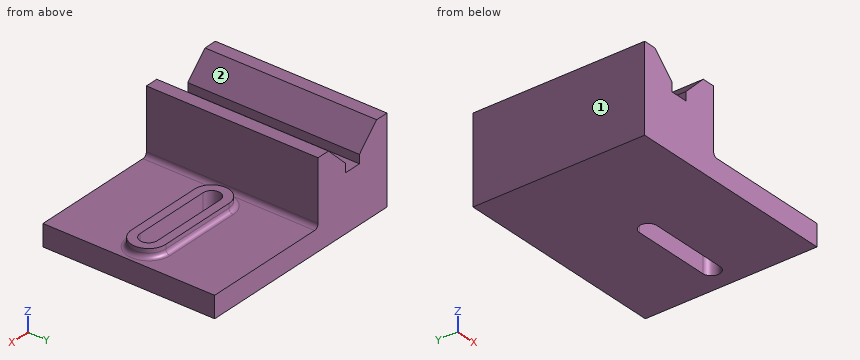
```python
from build123d import *

# Parameters (mm, degrees)
F1_DEPTH    = 200
F3_DEPTH    = 10
F4_DEPTH    = 25
F5_T1_DEPTH = 200
F5_T3_DEPTH = 91.5131680667
F5_T6_ANGLE = 180
F5_T8_ANGLE = 180


# Not quite as in the source:
# - a fillet or chamfer that OpenCascade refuses, or shapes differently, is made with other operations: its cross-section is extruded or revolved along the edge and cut away or added


with BuildPart() as f1:
    # F0 (on Front) → F1 (new body)
    with BuildSketch(Plane.XZ):
        Polygon((-250, 0), (0, 0), (0, 25), (-150, 25), (-150, 100), (-165, 100), (-190, 75), (-190, 65), (-210, 65), (-210, 75), (-235, 100), (-250, 100), align=None)
    extrude(amount=F1_DEPTH)

    # F2 (on face) → F3 (join)
    with BuildSketch(Plane.XY.offset(25)):
        with BuildLine():
            Line((-120.2453300357, -120), (-28.7321619689, -120))
            ThreePointArc((-28.7321619689, -120), (-8.7321619689, -100), (-28.7321619689, -80))
            Line((-28.7321619689, -80), (-120.2453300357, -80))
            ThreePointArc((-120.2453300357, -80), (-140.2453300357, -100), (-120.2453300357, -120))
        make_face()
        with BuildLine():
            ThreePointArc((-28.7321619689, -90), (-18.7321619689, -100), (-28.7321619689, -110))
            Line((-28.7321619689, -110), (-120.2453300357, -110))
            ThreePointArc((-120.2453300357, -110), (-130.2453300357, -100), (-120.2453300357, -90))
            Line((-120.2453300357, -90), (-28.7321619689, -90))
        make_face(mode=Mode.SUBTRACT)
    extrude(amount=F3_DEPTH)

    # F4 (cut): a face of the model
    f4_faces = [f1.faces().sort_by_distance(p)[0] for p in [
        (-74.4887460023, -100, 25),
    ]]
    extrude(f4_faces, amount=-F4_DEPTH, mode=Mode.SUBTRACT)

    # F5: fillet of radius 5 on 3 edges, made by hand

    # F5_s2 → F5_t1 (join)
    with BuildSketch(Plane.XZ):
        with BuildLine():
            ThreePointArc((-145, 25), (-148.5355339059, 26.4644660941), (-150, 30))
            Line((-150, 30), (-150, 25))
            Line((-150, 25), (-145, 25))
        make_face()
    extrude(amount=F5_T1_DEPTH)

    # F5_s4 → F5_t3 (join)
    with BuildSketch(Plane.YZ.offset(-120.2453300357)):
        with BuildLine():
            ThreePointArc((-125, 25), (-121.4644660941, 26.4644660941), (-120, 30))
            Line((-120, 30), (-120, 25))
            Line((-120, 25), (-125, 25))
        make_face()
        with BuildLine():
            ThreePointArc((-75, 25), (-78.5355339059, 26.4644660941), (-80, 30))
            Line((-80, 30), (-80, 25))
            Line((-80, 25), (-75, 25))
        make_face()
    extrude(amount=F5_T3_DEPTH)

    # F5_s5 → F5_t6 (revolve)
    with BuildSketch(Plane.YZ.offset(-28.7321619689)):
        with BuildLine():
            ThreePointArc((-120, 30), (-121.4644660941, 26.4644660941), (-125, 25))
            Line((-125, 25), (-120, 25))
            Line((-120, 25), (-120, 30))
        make_face()
    revolve(axis=Axis((-28.7321619689, -100, 25), (0, 0, 1)), revolution_arc=F5_T6_ANGLE)

    # F5_s7 → F5_t8 (revolve)
    with BuildSketch(Plane.YZ.offset(-120.2453300357)):
        with BuildLine():
            ThreePointArc((-75, 25), (-78.5355339059, 26.4644660941), (-80, 30))
            Line((-80, 30), (-80, 25))
            Line((-80, 25), (-75, 25))
        make_face()
    revolve(axis=Axis((-120.2453300357, -100, 25), (0, 0, 1)), revolution_arc=F5_T8_ANGLE)


solid = f1.part
```
Can you work these out from the model? Positions are in its coordinate system, mm. Face numbers are marked on the shaded views. A direction names the side the tool comes from. Give positions to 0.01 mm unless a question says otherwise; leave off trailing zeros. Loops run counter-clockwise (first coordinate to the right, second up) from the corner with the lowest first, then second, coordinate; pieces in that order, holes last. Notation, with made-up numbers: M 58,-31 L 85,-31 A18 cw 85,-20 Z; hole C 25,20 d11. An arc over 180 degrees is marked long. Use CSV: the item, a comma, the result in double quotes. Start each with the question number.
1. If I drill on L1, parallel to X at y = -85.5, z = 70; L2, parallel to X at y = -101, z = 32.5; L3, parallel to Z at x = -24.5, y = -63.5, over which ranges is the centre line in solid material (lowest first)?
2. On a 3-axis mill with a long thin cutter (end or side, diameter ignored), from which of +Z, -Z, +X, -X, +Y, -Y can I reach the whole of each face in a straight line? I mean the marked faces 1 and 2. Say none if no direction works.
3. Imagine slicing it at D-D, the plane z = 83.5. Write out the boundary of the cut face in (x, y).
4. Imagine slicing it at B-B, the plane x = -46. Write out the boundary of the cut face in (y, z), plus the area to 3 significant figures.
5. Imagine slicing it at C-C, the plane y = -100. Write out the boundary of the cut face in (x, z), plus the area to 3 significant figures.
6. For P1, Ø3, axis at y = -28, z = 58.5, coming from the +X side; P2, Ø6, axis at x = -28, y = -175.5, coming from the +Z side; P3, Ø16, axis at x = -199.5, y = -99, coming from the +Z side; P4, Ø10.5, axis at x = -96.5, z = 22, coming from the +Y side, each with a flat end and sliding along its axis, tell me the tip position at first contact or that it passes through.
7. Imagine slicing it at A-A, the plane z = 13. Write out the boundary of the cut face in (x, y).
Response values:
1,L1,"-250 to -210, -190 to -150"
1,L2,"-250 to -150, -140.22 to -130.2, -18.78 to -8.76"
1,L3,"0 to 25"
2,face 1,"+Z, -Z, -X, +Y, -Y"
2,face 2,"+Z, +Y, -Y"
3,outline,"M -250,-200 L -218.5,-200 L -218.5,0 L -250,0 Z; M -181.5,-200 L -150,-200 L -150,0 L -181.5,0 Z"
4,outline,"M -200,0 L -110,0 L -110,35 L -120,35 L -120,30 A5 cw -125,25 L -200,25 Z; M -90,0 L 0,0 L 0,25 L -75,25 A5 cw -80,30 L -80,35 L -90,35 Z"
4,area,"4,710 mm^2"
5,outline,"M -250,0 L -130.25,0 L -130.25,35 L -140.25,35 L -140.25,30 A5 cw -145.12,25 A5 cw -150,30 L -150,100 L -165,100 L -190,75 L -190,65 L -210,65 L -210,75 L -235,100 L -250,100 Z; M -18.73,0 L 0,0 L 0,25 L -3.73,25 A5 cw -8.73,30 L -8.73,35 L -18.73,35 Z"
5,area,"9,850 mm^2"
6,P1,"x = -150"
6,P2,"z = 25"
6,P3,"z = 65"
6,P4,"y = 0"
7,outline,"M -250,-200 L 0,-200 L 0,0 L -250,0 Z; hole M -120.25,-110 L -28.73,-110 A10 ccw -28.73,-90 L -120.25,-90 A10 ccw Z"
